```python
from build123d import *

# Parameters (mm, degrees)
CROQUIS1_W              = 6.56
CROQUIS1_H              = 2.56
SALIENTE_EXTRUIR1_DEPTH = 3


with BuildPart() as part:
    # Croquis1 → Saliente-Extruir1 (new body)
    # profile 1 of 4: a face of its own
    with BuildSketch(Plane.XY):
        with BuildLine():
            ThreePointArc((-6.599663594, -2.333332476), (-4.473021287, -12.08145136), (0, -21))
            ThreePointArc((0, -21), (7, -14), (14, -21))
            ThreePointArc((14, -21), (12.507710809, -9.830763064), (7, 0))
            ThreePointArc((7, 0), (-1.183713403, 6.899189994), (-6.599663594, -2.333332476))
        make_face()
        with Locations((0.22, 0.22)):
            Rectangle(CROQUIS1_W, CROQUIS1_H, mode=Mode.SUBTRACT)
    # profile 2 of 4: a face of its own
    with BuildSketch(Plane.XY):
        with BuildLine():
            ThreePointArc((14, -21), (7, -14), (0, -21))
            Line((0, -21), (14, -21))
        make_face()
    # profile 3 of 4: a face of its own
    with BuildSketch(Plane.XY):
        with BuildLine():
            Line((14, -21), (0, -21))
            ThreePointArc((0, -21), (4.213945985, -27.421674472), (11.782258008, -26.111751984))
            ThreePointArc((11.782258008, -26.111751984), (13.070021332, -23.633488722), (14, -21))
        make_face()
    # profile 4 of 4: a face of its own
    with BuildSketch(Plane.XY):
        with BuildLine():
            Line((-7.131748217, -35), (-3.131748217, -35))
            Line((-3.131748217, -35), (-3.131748217, -28))
            Line((-3.131748217, -28), (-0.131748217, -28))
            Line((-0.131748217, -28), (-0.131748217, -35))
            ThreePointArc((-0.131748217, -35), (6.681647081, -31.703803211), (11.782258008, -26.111751984))
            ThreePointArc((11.782258008, -26.111751984), (4.213945985, -27.421674472), (0, -21))
            ThreePointArc((0, -21), (-4.430558492, -27.559520621), (-7.131748217, -35))
        make_face()
    extrude(amount=SALIENTE_EXTRUIR1_DEPTH)


solid = part.part
```
Input: part model. Units: mm. Frame: model coordinates. A direction names the side the tool comes from. Give positions to 0.01 mm unless a question says otherwise; leave off trailing zeros. Order: outer loops, then holes, each group sorted by start corner. A loop starts at its lowest first (then second) coordinate and runs counter-clockwise, first axis right, second up. Notation, with made-up numbers: (-0.5, -25.5) - (3.5, -25.5) arc R21 ccw to (3.5, 11.5) - close; hole circle Ø8 at (69.25, -28). An arc over 180 degrees is marked (long way). Use a Markdown table: item, result.
(1) Pin query (flat end, axial travel): pin 1 (2 mm diameter, centred on x = 2, y = 0, fed in from +Z); pin 2 (1.3 mm diameter, centred on y = 0, z = 1.5, fed in from +X); pin 3 (0.9 mm diameter, centred on y = -31, z = 1.5, fed in from -X); pin 4 (1.5 mm diameter, centred on x = -1, z = 2, fed in from -Y). Return the tip coordinate at first contact, or that it passes through.
Computed values:
| item | result |
|---|---|
| pin 1 | passes through |
| pin 2 | stops at x = 7.53 |
| pin 3 | stops at x = -6.1 |
| pin 4 | stops at y = -28 |
(2) Section query B-B (x = 3). Output: boundary loops of the cut face in (y, z).
Computed values:
| item | result |
|---|---|
| outline | (-33.88, 0) - (-1.06, 0) - (-1.06, 3) - (-33.88, 3) - close; (1.5, 0) - (6.32, 0) - (6.32, 3) - (1.5, 3) - close |
(3) Section query D-D (y = -3.5). Output: boundary loops of the cut face in (x, z).
Computed values:
| item | result |
|---|---|
| outline | (-6.48, 0) - (9.54, 0) - (9.54, 3) - (-6.48, 3) - close |
(4) Section query C-C (y = -31). Output: boundary loops of the cut face in (x, z).
Computed values:
| item | result |
|---|---|
| outline | (-5.94, 0) - (-3.13, 0) - (-3.13, 3) - (-5.94, 3) - close; (-0.13, 0) - (7.57, 0) - (7.57, 3) - (-0.13, 3) - close |
(5) Access query for faces 1 (the cylindrical face through (-4.52, -11.95, 1.48)), 2 (the flat face through (-3.132, -32, 1)), 3 (the flat face through (0, -1.06, 1)). Directions: +Z, -Z, +X, -X, +Y, -Y. A direction counts if a zero-diameter tool reaches every point of the face in a straight line with its end or side. Return the directions, or none.
Computed values:
| item | result |
|---|---|
| face 1 | +Z, -Z, -X |
| face 2 | +Z, -Z, -Y |
| face 3 | +Z, -Z |
(6) Draft query along X for faces 4 (the cylindrical face through (-1.015, 6.926, 1.479)), 5 (the flat face through (-2, -28, 1)), 6 (the cylindrical face through (12.557, -9.981, 1.479)). Return one class per face: released by +X, released by -X, zero draft, split by the parting line, or undercut.
Computed values:
| item | result |
|---|---|
| face 4 | split by the parting line |
| face 5 | undercut |
| face 6 | released by +X |
(7) Section query A-A (z = 2.25). Output: boundary loops of the cut face in (x, y), then the cut area to 3 significant figures.
Computed values:
| item | result |
|---|---|
| outline | (-7.13, -35) - (-3.13, -35) - (-3.13, -28) - (-0.13, -28) - (-0.13, -35) arc R20 ccw to (14, -21) arc R30 ccw to (7, 0) arc R7 ccw (long way) to (-6.6, -2.33) arc R40 ccw to (0, -21) arc R32.28 ccw to start; hole (-3.06, -1.06) - (3.5, -1.06) - (3.5, 1.5) - (-3.06, 1.5) - close |
| area | 578 mm2 |
(8) Line query: line 1 (Y direction, x = -1.5, z = 0.7); line 2 (Y direction, x = -1.25, z = 2.2); line 3 (X direction, y = 0.5, z = 2.4). Output: solid intervals per line, ascending. Write a range as from..to.
Computed values:
| item | result |
|---|---|
| line 1 | y = -28..-22.85, -18.58..-1.06, 1.5..6.84 |
| line 2 | y = -28..-22.53, -19.01..-1.06, 1.5..6.89 |
| line 3 | x = -6.98..-3.06, 3.5..6.98 |
